Here's how the part is built. I have some questions about the finished solid (model axes, mm). Face numbers are marked on the shaded views. A direction names the side the tool comes from. Round coordinates to 2 decimals unless told otherwise and drop trailing zeros. Write each loop counter-clockwise with the first axis right and the second up, starting at its lowest first coordinate (ties: lowest second). Pieces come first, ordered by that corner, then holes. Notation, with made-up numbers: (56.25, -28.5) -> (111.25, -28.5) arc R18 ccw to (111.25, -0.5) -> close; hole circle Ø5 at (-39.5, -35.5). An arc over 180 degrees is marked (long way). Put each result on its own line as item: value. Start each with the question number.
1. Which directions (+Z, -Z, +X, -X, +Y, -Y) give clear straight access to the entire face, cutting with the end or side of a thin tool? Please do the marked faces 1, 2, 3, 4 and 5.
2. Suppose I cut it at A-A (y = 9). Please give me the cut outline in (x, z).
3. I need wall thicknesses on probe 1 along X at (y, z) = (-2.5, 8.5); probe 2 along Z at (x, y) = (-44, -20.5); probe 3 along Z at (x, y) = (-53.5, 6). Which ranges of each line are inside material? Lowest first, please. Write a range as from..to.
4. We'd pull the mould along Y, two halves only. Please class the marked faces 6, 7 and 8: +Y half, -Y half, draft (parallel to the pull), parting line (faces both ways), or undercut.
5. For pin 1 (1.5 mm diameter, centred on y = -21.5, z = -9.5, fed in from -X); pin 2 (11 mm diameter, centred on y = -21, z = -0.5, fed in from -X); pin 3 (5 mm diameter, centred on y = -19, z = -2.5, fed in from -X); pin 4 (17.5 mm diameter, centred on x = -30, y = 4.5, fed in from -Z), each with a flat end and sliding along its axis, tell me the tip position at first contact or that it passes through.
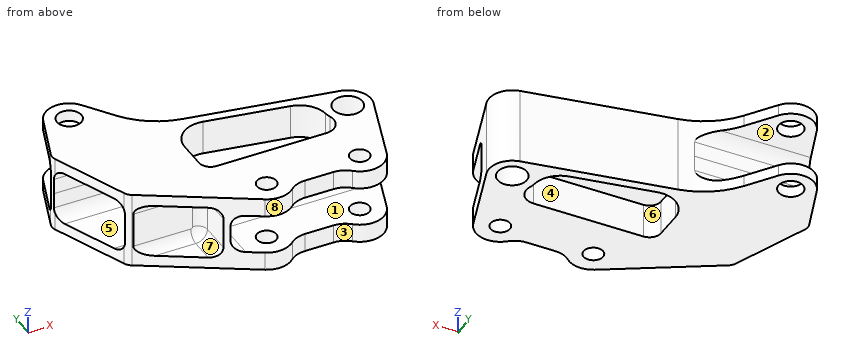
```python
from build123d import *

# Parameters (mm, degrees)
SKETCH1_R           = 4.7625
SKETCH1_R_2         = 4
SKETCH1_R_3         = 3.175
BOSS_EXTRUDE1_DEPTH = 12.573
BOSS_EXTRUDE2_DEPTH = 1.27
SKETCH1_6_R         = 3.175
CUT_EXTRUDE1_DEPTH  = 6.477
SKETCH1_10_R        = 4
CUT_EXTRUDE3_DEPTH  = 8.89
FILLET1_R           = 3.81
FILLET3_R           = 3.81
FILLET4_R           = 3.175
FILLET5_R           = 7.62


with BuildPart() as part:
    # Sketch1 → Boss-Extrude1 (new body)
    with BuildSketch(Plane(origin=(0, 0, 0), x_dir=(0, 1, 0), z_dir=(0, 0, 1))):
        with BuildLine():
            Line((-26.499431941, 0.950631657), (-2.449998994, -7.215393609))
            ThreePointArc((-2.449998994, -7.215393609), (3.866048142, -6.56643524), (7.497932311, -1.358459074))
            Line((7.497932311, -1.358459074), (16.069122988, 45.94970705))
            ThreePointArc((16.069122988, 45.94970705), (19.672222889, 55.119231342), (26.493389209, 62.227972063))
            Line((26.493389209, 62.227972063), (35.774163974, 68.726440514))
            ThreePointArc((35.774163974, 68.726440514), (38.958321373, 75.962988676), (34.009705021, 82.128836862))
            Line((34.009705021, 82.128836862), (16.544511529, 88.485647429))
            Line((16.544511529, 88.485647429), (-10.358349656, 77.508379092))
            Line((-10.358349656, 77.508379092), (-30.779024566, 42.987968953))
            ThreePointArc((-30.779024566, 42.987968953), (-31.601546647, 36.844959103), (-27.757349656, 31.983348043))
            Line((-27.757349656, 31.983348043), (-27.757349656, 15.42998529))
            ThreePointArc((-27.757349656, 15.42998529), (-31.855063811, 7.779670964), (-26.499431941, 0.950631657))
        make_face()
        with Locations(Location((0, 0, 0), (0, 0, 270))):
            Circle(SKETCH1_R, mode=Mode.SUBTRACT)
        with Locations(Location((31.403511529, 74.968379092, 0), (0, 0, 270))):
            Circle(SKETCH1_R_2, mode=Mode.SUBTRACT)
        with Locations(Location((-23.947349656, 38.946666667, 0), (0, 0, 270))):
            Circle(SKETCH1_R_3, mode=Mode.SUBTRACT)
        with Locations(Location((-23.947349656, 8.466666667, 0), (0, 0, 270))):
            Circle(SKETCH1_R_3, mode=Mode.SUBTRACT)
        with BuildLine():
            Line((-9.469349656, 47.836666667), (-9.469349656, 11.917365883))
            ThreePointArc((-9.469349656, 11.917365883), (-7.295140555, 7.750499045), (-2.633609794, 7.15041953))
            ThreePointArc((-2.633609794, 7.15041953), (-1.656512431, 7.437766235), (-0.649822418, 7.592241489))
            ThreePointArc((-0.649822418, 7.592241489), (4.576435948, 9.875722251), (7.339639123, 14.86498764))
            Line((7.339639123, 14.86498764), (12.10584978, 41.171797748))
            ThreePointArc((12.10584978, 41.171797748), (10.181808987, 48.455026751), (3.358262084, 51.646666667))
            Line((3.358262084, 51.646666667), (-5.659349656, 51.646666667))
            ThreePointArc((-5.659349656, 51.646666667), (-8.353426493, 50.530743503), (-9.469349656, 47.836666667))
        make_face(mode=Mode.SUBTRACT)
    extrude(amount=BOSS_EXTRUDE1_DEPTH)

    # Sketch1<4> → Boss-Extrude2 (add)
    with BuildSketch(Plane(origin=(0, 0, 0), x_dir=(0, 1, 0), z_dir=(0, 0, 1))):
        with BuildLine():
            ThreePointArc((-5.659349656, 51.646666667), (-8.353426493, 50.530743503), (-9.469349656, 47.836666667))
            Line((-9.469349656, 47.836666667), (-9.469349656, 11.917365883))
            ThreePointArc((-9.469349656, 11.917365883), (-7.295140555, 7.750499045), (-2.633609794, 7.15041953))
            ThreePointArc((-2.633609794, 7.15041953), (-1.656512431, 7.437766235), (-0.649822418, 7.592241489))
            ThreePointArc((-0.649822418, 7.592241489), (4.576435948, 9.875722251), (7.339639123, 14.86498764))
            Line((7.339639123, 14.86498764), (12.10584978, 41.171797748))
            ThreePointArc((12.10584978, 41.171797748), (10.181808987, 48.455026751), (3.358262084, 51.646666667))
            Line((3.358262084, 51.646666667), (-5.659349656, 51.646666667))
        make_face()
    extrude(amount=BOSS_EXTRUDE2_DEPTH)

    # Sketch1<6> → Cut-Extrude1 (cut)
    with BuildSketch(Plane(origin=(0, 0, 0), x_dir=(0, 1, 0), z_dir=(0, 0, 1))):
        with BuildLine():
            ThreePointArc((-27.757349656, 15.42998529), (-31.855063811, 7.779670964), (-26.499431941, 0.950631657))
            Line((-26.499431941, 0.950631657), (-11.247349656, -4.228238446))
            Line((-11.247349656, -4.228238446), (-11.247349656, 51.646666667))
            Line((-11.247349656, 51.646666667), (-25.656940256, 51.646666667))
            Line((-25.656940256, 51.646666667), (-30.779024566, 42.987968953))
            ThreePointArc((-30.779024566, 42.987968953), (-31.601546647, 36.844959103), (-27.757349656, 31.983348043))
            Line((-27.757349656, 31.983348043), (-27.757349656, 15.42998529))
        make_face()
        with Locations(Location((-23.947349656, 8.466666667, 0), (0, 0, 270))):
            Circle(SKETCH1_6_R, mode=Mode.SUBTRACT)
        with Locations(Location((-23.947349656, 38.946666667, 0), (0, 0, 270))):
            Circle(SKETCH1_6_R, mode=Mode.SUBTRACT)
    extrude(amount=CUT_EXTRUDE1_DEPTH, mode=Mode.SUBTRACT)

    # Sketch1<10> → Cut-Extrude3 (cut)
    # profile 1 of 3: a face of its own
    with BuildSketch(Plane(origin=(0, 0, 0), x_dir=(0, 1, 0), z_dir=(0, 0, 1))):
        with BuildLine():
            Line((17.433511529, 88.162077891), (17.433511529, 50.740503147))
            ThreePointArc((17.433511529, 50.740503147), (21.118462359, 57.150658387), (26.493389209, 62.227972063))
            Line((26.493389209, 62.227972063), (35.774163974, 68.726440514))
            ThreePointArc((35.774163974, 68.726440514), (38.958321373, 75.962988676), (34.009705021, 82.128836862))
            Line((34.009705021, 82.128836862), (17.433511529, 88.162077891))
        make_face()
        with Locations(Location((31.403511529, 74.968379092, 0), (0, 0, 270))):
            Circle(SKETCH1_10_R, mode=Mode.SUBTRACT)
    # profile 2 of 3: a face of its own
    with BuildSketch(Plane(origin=(0, 0, 0), x_dir=(0, 1, 0), z_dir=(0, 0, 1))):
        Polygon((-11.247349656, 76.005556842), (-24.605157851, 53.424666667), (-11.247349656, 53.424666667), align=None)
    # profile 3 of 3: a face of its own
    with BuildSketch(Plane(origin=(0, 0, 0), x_dir=(0, 1, 0), z_dir=(0, 0, 1))):
        Polygon((15.655511529, 88.122905656), (-9.469349656, 77.871120864), (-9.469349656, 53.424666667), (15.655511529, 53.424666667), align=None)
    extrude(amount=CUT_EXTRUDE3_DEPTH, mode=Mode.SUBTRACT)

    # Mirror1: part across face


with BuildPart() as part_1:
    add(part.part)
    add(part.part.mirror(Plane(origin=(-30.744300958, 0.707665305, 0), x_dir=(1, 0, 0), z_dir=(0, 0, -1))))

    # Fillet1
    fillet1_edges = [part_1.edges().sort_by_distance(p)[0] for p in [
        (-69.451290519, 17.433511529, 8.89),
        (-51.646666667, -18.452144956, 6.477),
        (-51.646666667, -18.452144956, -6.477),
        (-53.424666667, -17.926253754, 8.89),
        (-53.424666667, -17.926253754, -8.89),
        (-70.773786162, 15.655511529, 8.89),
        (-65.647893765, -9.469349656, 8.89),
        (-65.647893765, -9.469349656, -8.89),
        (-70.773786162, 15.655511529, -8.89),
        (-69.451290519, 17.433511529, -8.89),
    ]]
    fillet(fillet1_edges, radius=FILLET1_R)

    # Fillet3
    # the kernel refuses this fillet: 3.81 mm, written as the material it takes off along each edge
    with BuildSketch(Plane(origin=(-77.508379092, -10.358349656, -15.77817458), x_dir=(-0.3777939966211631, 0.9258896781566412, 0), z_dir=(0, 0, 1))) as fillet3_piece_1:
        with BuildLine():
            CenterArc((FILLET3_R * 0.336501268256, -FILLET3_R), FILLET3_R, 90, 37.196303294)
            Line((-FILLET3_R * 0.268046453486, -FILLET3_R * 0.203431075087), (0, 0))
            Line((0, 0), (FILLET3_R * 0.336501268256, 0))
        make_face()
    extrude(amount=31.55634916, mode=Mode.SUBTRACT)
    with BuildSketch(Plane(origin=(-88.485647429, 16.544511529, -16.248115103), x_dir=(0.3420201433256622, 0.9396926207859108, 0), z_dir=(0, 0, 1))) as fillet3_piece_2:
        with BuildLine():
            CenterArc((FILLET3_R * 0.385838855973, -FILLET3_R), FILLET3_R, 90, 42.197104506)
            Line((-FILLET3_R * 0.285844295256, -FILLET3_R * 0.259161458646), (0, 0))
            Line((0, 0), (FILLET3_R * 0.385838855973, 0))
        make_face()
    extrude(amount=32.496230206, mode=Mode.SUBTRACT)

    # Fillet4
    fillet4_edges = [part_1.edges().sort_by_distance(p)[0] for p in [
        (-53.424666667, -11.247349656, 0),
        (-66.620111754, -11.247349656, -8.89),
        (-66.620111754, -11.247349656, 8.89),
        (-54.54058983, -11.247349656, -7.774076836),
        (-54.54058983, -11.247349656, 7.774076836),
        (-21.80421411, -11.247349656, 6.477),
        (-51.646666667, -11.247349656, 0),
        (-21.80421411, -11.247349656, -6.477),
        (-50.530743503, -11.247349656, -5.361076836),
        (-50.530743503, -11.247349656, 5.361076836),
    ]]
    fillet(fillet4_edges, radius=FILLET4_R)

    # Fillet5
    fillet5_edges = [part_1.edges().sort_by_distance(p)[0] for p in [
        (-31.983348043, -27.757349656, -9.525),
        (-15.42998529, -27.757349656, -9.525),
        (-15.42998529, -27.757349656, 9.525),
        (-31.983348043, -27.757349656, 9.525),
    ]]
    fillet(fillet5_edges, radius=FILLET5_R)


solid = part_1.part
```
Verdict:
1. face 1: +X, -Y
1. face 2: +X, -X, +Y
1. face 3: +Z, -Z, -Y
1. face 4: -Z
1. face 5: -X
2. outline: (-85.41, -12.57) -> (-49.63, -12.57) -> (-49.63, -1.27) -> (-24.03, -1.27) -> (-24.03, -12.57) -> (-6.93, -12.57) -> (-6.93, 12.57) -> (-24.03, 12.57) -> (-24.03, 1.27) -> (-49.63, 1.27) -> (-49.63, 12.57) -> (-85.41, 12.57) -> (-85.41, 8.89) -> (-53.42, 8.89) -> (-53.42, -8.89) -> (-85.41, -8.89) -> close
3. probe 1: x = -53.42..-51.65, -7.2..-4.05, 4.05..7.2
3. probe 2: z = -12.57..-6.48, 6.48..12.57
3. probe 3: z = -12.57..-8.89, 8.89..12.57
4. face 6: undercut
4. face 7: draft
4. face 8: -Y half
5. pin 1: stops at x = -59.94
5. pin 2: stops at x = -53.54
5. pin 3: stops at x = -53.42
5. pin 4: stops at z = -12.57
